from build123d import *

# Parameters (mm, degrees)
SKETCH_1_W          = 40
SKETCH_1_H          = 41
EXTRUDE_1_DEPTH     = 20
SKETCH_2_R          = 6
EXTRUDE_2_DEPTH     = 2
SKETCH_3_R          = 2.5
EXTRUDE_3_DEPTH     = 5.1
SKETCH_4_W          = 2.5
SKETCH_4_H          = 20
EXTRUDE_4_DEPTH     = 7.25
SKETCH_5_R          = 3
CUT_EXTRUDE_2_DEPTH = 2.5


with BuildPart() as part:
    # 草图1 → 凸台-拉伸1 (new body)
    with BuildSketch(Plane(origin=(0, 0, 0), x_dir=(1, 0, 0), z_dir=(0, 1, 0))):
        with Locations((20, 20.5)):
            Rectangle(SKETCH_1_W, SKETCH_1_H)
    extrude(amount=EXTRUDE_1_DEPTH)

    # 草图2 → 凸台-拉伸2 (add)
    with BuildSketch(Plane.XY):
        with Locations((30, 10)):
            Circle(SKETCH_2_R)
    extrude(amount=EXTRUDE_2_DEPTH)

    # 草图3 → 凸台-拉伸3 (add)
    with BuildSketch(Plane.XY.offset(2)):
        with Locations((30, 10)):
            Circle(SKETCH_3_R)
    extrude(amount=EXTRUDE_3_DEPTH)

    # 草图4 → 凸台-拉伸4 (add)
    with BuildSketch(Plane.ZY):
        with Locations((-7.05, 10)):
            Rectangle(SKETCH_4_W, SKETCH_4_H)
    extrude_4 = extrude(amount=EXTRUDE_4_DEPTH)

    # 草图5 → 切除-拉伸2 (cut)
    with BuildSketch(Plane.XY.offset(-5.8)):
        with Locations((-4.75, 15)):
            Circle(SKETCH_5_R)
        with Locations((-4.75, 5)):
            Circle(SKETCH_5_R)
    cut_extrude_2 = extrude(amount=-CUT_EXTRUDE_2_DEPTH, mode=Mode.SUBTRACT)

    # 镜向1: 凸台-拉伸4, 切除-拉伸2 across plane
    add(extrude_4.mirror(Plane.ZY.offset(-20)))
    add(cut_extrude_2.mirror(Plane.ZY.offset(-20)), mode=Mode.SUBTRACT)


solid = part.part
Could you check a few things on this model? Use its own coordinates, in mm. A direction names the side the tool comes from. Give positions to 0.01 mm unless a question says otherwise; leave off trailing zeros. Order: outer loops, then holes, each group sorted by start corner. A loop starts at its lowest first (then second) coordinate and runs counter-clockwise, first axis right, second up. Notation, with made-up numbers: (60.5, 70) - (73.5, 70) arc R25 cw to (73.5, 108) - close; hole circle Ø4 at (72.25, 6.5). An arc over 180 degrees is marked (long way). Return JSON: item names as keys, results as strings. Group by question number.
Q1. Suppose I cut it at A-A, the plane x = -4.75. Please give me the cut outline in (y, z), and give its area (3 significant figures).
Q2. Which directions (+Z, -Z, +X, -X, +Y, -Y) give clear straight access to the entire face, cutting with the end or side of a thin tool? Please do faces 5 (the face through (43, 10, -5.8)), 6 (the face through (-3, 10, -8.3)), 7 (the face through (25.24, 6.35, 0.99)), 8 (the face through (40, 10, -24)).
Q3. Thinking about a two-plate mould opening in Y: for faces 1 (the face through (41.752, 4.893, -7.033)), 2 (the face through (47.25, 10, -7)), 3 (the face through (29.46, 7.56, 4.51)), 4 (the face through (-1.752, 4.893, -7.033)), which applies, pulls with the +Y half, pulls with the -Y half, needs draft (parallel to the pull), parting line crosses it, or undercut?
Q4. Will these pins go through, and if not, where does the flat tip stop? pin 1 Ø12 at (y, z) = (17, -25.5) entering from -X; pin 2 Ø8 at (x, y) = (44.5, 13) entering from -Z; pin 3 Ø10 at (y, z) = (13.5, -34) entering from +X; pin 4 Ø5 at (x, y) = (-4.75, 15) entering from -Z.
Q5. Suppose I cut it at C-C, the plane x = 30. Please give me the cut outline in (y, z), and give its area (4 significant figures).
Q6. Please list where these lines run through material, in increasing order: line 1 along Y through (x, z) = (-4.75, -6.85); line 2 along Y through (x, z) = (44, -7); line 3 along X through (y, z) = (15, -7.05). Write a range as [from, to].
Q7. Suppose I cut it at B-B, the plane y = 10. Please give me the cut outline in (x, z), and give its area (3 significant figures).
Q8. Suppose I cut it at D-D, the plane z = -34. Please give me the cut outline in (x, y), and give its area (3 significant figures).
Resolved:
{
 "1": {"outline": "(0, -8.3) - (2, -8.3) - (2, -5.8) - (0, -5.8) - close; (8, -8.3) - (12, -8.3) - (12, -5.8) - (8, -5.8) - close; (18, -8.3) - (20, -8.3) - (20, -5.8) - (18, -5.8) - close", "area": "20.0 mm2"},
 "2": {"face 5": "+Z, +X, +Y, -Y", "face 6": "-Z, -X, +Y, -Y", "face 7": "+Z", "face 8": "-Z, +X, +Y, -Y"},
 "3": {"face 1": "undercut", "face 2": "needs draft", "face 3": "parting line crosses it", "face 4": "undercut"},
 "4": {"pin 1": "stops at x = 0", "pin 2": "stops at z = -8.3", "pin 3": "stops at x = 40", "pin 4": "passes through"},
 "5": {"outline": "(0, -41) - (20, -41) - (20, 0) - (16, 0) - (16, 2) - (12.5, 2) - (12.5, 7.1) - (7.5, 7.1) - (7.5, 2) - (4, 2) - (4, 0) - (0, 0) - close", "area": "869.5 mm2"},
 "6": {"line 1": "y = [0, 2], [8, 12], [18, 20]", "line 2": "y = [0, 2.1], [7.9, 12.1], [17.9, 20]", "line 3": "x = [-1.75, 41.75]"},
 "7": {"outline": "(-7.25, -8.3) - (0, -8.3) - (0, -41) - (40, -41) - (40, -8.3) - (47.25, -8.3) - (47.25, -5.8) - (40, -5.8) - (40, 0) - (36, 0) - (36, 2) - (32.5, 2) - (32.5, 7.1) - (27.5, 7.1) - (27.5, 2) - (24, 2) - (24, 0) - (0, 0) - (0, -5.8) - (-7.25, -5.8) - close", "area": "1,730 mm2"},
 "8": {"outline": "(0, 0) - (40, 0) - (40, 20) - (0, 20) - close", "area": "800 mm2"}
}
